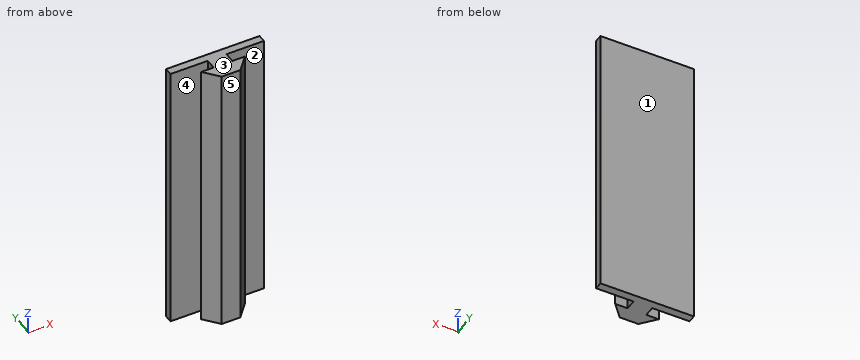
Autodesk Inventor part; units mm, degrees
ref_plane "YZ Plane" through (0, 0, 0) normal (1, 0, 0) x (0, 1, 0)
ref_plane "XZ Plane" through (0, 0, 0) normal (0, 1, 0) x (-1, 0, 0)
ref_plane "XY Plane" through (0, 0, 0) normal (0, 0, 1) x (1, 0, 0)
sketch "Sketch1" plane through (0, 0, 0) normal (0, 1, 0) x (-1, 0, 0)
  line L0 (0, 0) -> (38.1, 0)
  line L1 (38.1, 0) -> (38.1, -114.3)
  line L2 (38.1, -114.3) -> (0, -114.3)
  line L3 (0, -114.3) -> (0, 0)
  dimension "d0" = 38.1
  dimension "d1" = 114.3
extrude "Extrusion1" add sketch "Sketch1" along normal blind 3.175
sketch "Sketch2" plane through (-38.1, 0, 0) normal (0, 0, 1) x (1, 0, 0)
  line L0 (38.1, 0) -> (0, 0)
  line L1 (15.24, 0) -> (15.24, -4.318)
  line L2 (22.86, -4.318) -> (22.86, 0)
  line L3 (15.24, 0) -> (22.86, 0)
  line L4 (0, 0) -> (0, 3.175)
  line L5 (38.1, 0) -> (38.1, 3.175)
  line L6 (22.86, -4.318) -> (27.94, -4.318)
  line L7 (15.24, -4.318) -> (10.16, -4.318)
  line L8 (10.16, -4.318) -> (15.24, -10.16)
  line L9 (15.24, -10.16) -> (22.86, -10.16)
  line L10 (22.86, -10.16) -> (27.94, -4.318)
  dimension "d4" = 15.24
  dimension "d5" = 15.24
  dimension "d7" = 5.08
  dimension "d8" = 5.08
  dimension "d9" = 7.62
  dimension "d10" = 10.16
extrude "Extrusion2" add sketch "Sketch2" against normal blind 114.3
properties part number "railMount_4.5inch"
Geometry: final body of the model. Coordinates: model frame, mm. Face numbers are marked on the shaded views. A direction names the side the tool comes from. Round coordinates to 2 decimals unless told otherwise and drop trailing zeros. Write each loop counter-clockwise with the first axis right and the second up, starting at its lowest first coordinate (ties: lowest second). Pieces come first, ordered by that corner, then holes. Notation, with made-up numbers: (6, -28) -> (28, -28) arc R8 ccw to (28, -14) -> close; hole circle Ø10 at (56, 65.5). An arc over 180 degrees is marked (long way). Return JSON: item names as keys, results as strings.
Q1. Section A-A on z = -104.5. Return the cut outline in (x, y) (3 decimals).
From the geometry:
{"outline": "(-38.1, 0) -> (-22.86, 0) -> (-22.86, -4.318) -> (-27.94, -4.318) -> (-22.86, -10.16) -> (-15.24, -10.16) -> (-10.16, -4.318) -> (-15.24, -4.318) -> (-15.24, 0) -> (0, 0) -> (0, 3.175) -> (-38.1, 3.175) -> close"}
Q2. Section D-D on x = -7. Return the cut outline in (y, z) (3 decimals), and give its area (3 significant figures).
From the geometry:
{"outline": "(0, -114.3) -> (3.175, -114.3) -> (3.175, 0) -> (0, 0) -> close", "area": "363 mm2"}
Q3. Ray query, line 1 (Y direction, x = -33, z = -93.5) (3 decimals); line 2 (Y direction, x = -25, z = -75.5) (3 decimals); line 3 (X direction, y = -2.5, z = -56). Return the intervals inside material, ascending.
From the geometry:
{"line 1": "0 to 3.175", "line 2": "-7.699 to -4.318, 0 to 3.175", "line 3": "-22.86 to -15.24"}
Q4. First-contact query: pin 1 Ø8 at (y, z) = (-6.5, -86.5) entering from +X; pin 2 Ø4.5 at (x, z) = (-26.5, -33.5) entering from -Y; pin 3 Ø1.5 at (x, y) = (-9, -5) entering from -Z; pin 4 Ø1.3 at (y, z) = (-3, -51) entering from -X. Flat tips, straight axial feed; report the tip coordinate or a pass-through.
From the geometry:
{"pin 1": "x = -10.16", "pin 2": "y = -8.56", "pin 3": "through", "pin 4": "x = -22.86"}
Q5. Set-up query: the marked faces 1 and 2. Return all of +Z, -Z, +X, -X, +Y, -Y with unobstructed straight access to the full face (end or side cutting, diameter ignored); none if empty.
From the geometry:
{"face 1": "+Z, -Z, +X, -X, +Y", "face 2": "+Z, -Z, +X"}
Q6. Section C-C on y = -1.25. Return the cut outline in (x, z), and give its area (3 significant figures).
From the geometry:
{"outline": "(-22.86, -114.3) -> (-15.24, -114.3) -> (-15.24, 0) -> (-22.86, 0) -> close", "area": "871 mm2"}
Q7. Section B-B on x = -25.5. Return the cut outline in (y, z) (3 decimals), and give its area (3 significant figures).
From the geometry:
{"outline": "(-7.124, -114.3) -> (-4.318, -114.3) -> (-4.318, 0) -> (-7.124, 0) -> close; (0, -114.3) -> (3.175, -114.3) -> (3.175, 0) -> (0, 0) -> close", "area": "684 mm2"}
Q8. Mould query, pull axis Y, two halves, no side actions, for the marked faces 3, 4 and 5. Classes: +Y half, -Y half, draft (parallel to the pull), parting line (faces both ways), or undercut.
From the geometry:
{"face 3": "draft", "face 4": "undercut", "face 5": "-Y half"}
